```python
from build123d import *

# Parameters (mm, degrees)
SKETCH2_W           = 57
SKETCH2_H           = 120.75
SKETCH2_W_2         = 51
SKETCH2_H_2         = 114.75
BOSS_EXTRUDE1_DEPTH = 75
SKETCH3_W           = 57
SKETCH3_H           = 120.75
BOSS_EXTRUDE2_DEPTH = 3
SKETCH4_W           = 78
SKETCH4_H           = 57
BOSS_EXTRUDE3_DEPTH = 5
SKETCH6_R           = 2.675
CUT_EXTRUDE2_DEPTH  = 10
CUT_EXTRUDE3_DEPTH  = 58
BOSS_EXTRUDE4_REACH = 59
CUT_EXTRUDE7_DEPTH  = 126.75
SKETCH18_R          = 1.75
SKETCH18_W          = 28.5
SKETCH18_H          = 55
CUT_EXTRUDE8_DEPTH  = 10
BOSS_EXTRUDE6_DEPTH = 5
CUT_EXTRUDE9_DEPTH  = 5
CHAMFER1_SIZE       = 2


with BuildPart() as part:
    # Sketch2 → Boss-Extrude1 (new body)
    with BuildSketch(Plane(origin=(0, 0, 0), x_dir=(0, 0, -1), z_dir=(1, 0, 0))):
        with Locations((2.896243414, -39.494242434)):
            Rectangle(SKETCH2_W, SKETCH2_H)
        with Locations((2.896243414, -39.494242434)):
            Rectangle(SKETCH2_W_2, SKETCH2_H_2, mode=Mode.SUBTRACT)
    extrude(amount=BOSS_EXTRUDE1_DEPTH)

    # Sketch3 → Boss-Extrude2 (add)
    with BuildSketch(Plane.ZY):
        with Locations((-2.896243414, -39.494242434)):
            Rectangle(SKETCH3_W, SKETCH3_H)
    extrude(amount=BOSS_EXTRUDE2_DEPTH)

    # Sketch4 → Boss-Extrude3 (add)
    with BuildSketch(Plane(origin=(0, 20.880757566, 0), x_dir=(1, 0, 0), z_dir=(0, 1, 0))):
        with Locations((36, 2.896243414)):
            Rectangle(SKETCH4_W, SKETCH4_H)
    extrude(amount=BOSS_EXTRUDE3_DEPTH)

    # Sketch6 → Cut-Extrude2 (cut)
    with BuildSketch(Plane(origin=(0, 25.880757566, 0), x_dir=(1, 0, 0), z_dir=(0, 1, 0))):
        with Locations((36, 18.896243414)):
            Circle(SKETCH6_R)
        with Locations((36, -13.103756586)):
            Circle(SKETCH6_R)
    extrude(amount=-CUT_EXTRUDE2_DEPTH, mode=Mode.SUBTRACT)

    # Sketch8 → Cut-Extrude3 (cut, through all)
    with BuildSketch(Plane(origin=(0, 0, -31.396243414), x_dir=(-1, 0, 0), z_dir=(0, 0, -1))):
        Polygon((3, -99.869242434), (3, -79.869242434), (-17, -99.869242434), align=None)
    extrude(amount=-CUT_EXTRUDE3_DEPTH, mode=Mode.SUBTRACT)

    # Sketch9 → Boss-Extrude4 (add, up to next)
    with BuildSketch(Plane.XY.offset(25.603756586), mode=Mode.PRIVATE) as boss_extrude4_sk1:
        Polygon((-3, -79.869242434), (17, -99.869242434), (21.242640687, -99.869242434), (-3, -75.626601747), align=None)
    boss_extrude4_tool1 = extrude(boss_extrude4_sk1.sketch, amount=-BOSS_EXTRUDE4_REACH, mode=Mode.PRIVATE) - part.part
    add(boss_extrude4_tool1.solids().sort_by_distance((8.094564, -88.774678, 25.603757))[0])

    # Sketch15 → Cut-Extrude7 (cut, through all)
    with BuildSketch(Plane.XZ.offset(99.869242434)):
        with BuildLine():
            Line((62.625, 7.226342188), (62.625, 11.976342188))
            ThreePointArc((62.625, 11.976342188), (65, 14.351342188), (67.375, 11.976342188))
            Line((67.375, 11.976342188), (67.375, 7.226342188))
            ThreePointArc((67.375, 7.226342188), (65, 4.851342188), (62.625, 7.226342188))
        make_face()
        with BuildLine():
            Line((62.625, -17.72757696), (62.625, -12.97757696))
            ThreePointArc((62.625, -12.97757696), (65, -10.60257696), (67.375, -12.97757696))
            Line((67.375, -12.97757696), (67.375, -17.72757696))
            ThreePointArc((67.375, -17.72757696), (65, -20.10257696), (62.625, -17.72757696))
        make_face()
    extrude(amount=-CUT_EXTRUDE7_DEPTH, mode=Mode.SUBTRACT)

    # Sketch18 → Cut-Extrude8 (cut)
    with BuildSketch(Plane.ZY.offset(3)):
        with Locations((-22.896243414, -14.119242434)):
            Circle(SKETCH18_R)
        with Locations((17.103756586, -14.119242434)):
            Circle(SKETCH18_R)
        with Locations((-2.896243414, -14.119242434)):
            Rectangle(SKETCH18_W, SKETCH18_H)
    extrude(amount=-CUT_EXTRUDE8_DEPTH, mode=Mode.SUBTRACT)

    # Sketch21 → Boss-Extrude6 (add)
    with BuildSketch(Plane(origin=(0, 0, 0), x_dir=(0, 0, -1), z_dir=(1, 0, 0))):
        with BuildLine():
            Line((22.896243414, -19.869242434), (28.646243414, -19.869242434))
            Line((28.646243414, -19.869242434), (28.646243414, -8.369242434))
            Line((28.646243414, -8.369242434), (22.896243414, -8.369242434))
            ThreePointArc((22.896243414, -8.369242434), (17.146243414, -14.119242434), (22.896243414, -19.869242434))
        make_face()
        Polygon((19.518744339, -14.119242434), (21.207493877, -11.194242434), (24.584992952, -11.194242434), (26.273742489, -14.119242434), (24.584992952, -17.044242434), (21.207493877, -17.044242434), align=None, mode=Mode.SUBTRACT)
        with BuildLine():
            Line((-17.103756586, -19.869242434), (-22.853756586, -19.869242434))
            Line((-22.853756586, -19.869242434), (-22.853756586, -8.369242434))
            Line((-22.853756586, -8.369242434), (-17.103756586, -8.369242434))
            ThreePointArc((-17.103756586, -8.369242434), (-11.353756586, -14.119242434), (-17.103756586, -19.869242434))
        make_face()
        Polygon((-15.415007048, -11.194242434), (-18.792506123, -11.194242434), (-20.481255661, -14.119242434), (-18.792506123, -17.044242434), (-15.415007048, -17.044242434), (-13.726257511, -14.119242434), align=None, mode=Mode.SUBTRACT)
    extrude(amount=BOSS_EXTRUDE6_DEPTH)

    # Sketch22 → Cut-Extrude9 (cut)
    with BuildSketch(Plane.XZ.offset(-17.880757566)):
        Polygon((40.820874748, -18.896243414), (38.410437374, -14.721243414), (33.589562626, -14.721243414), (31.179125252, -18.896243414), (33.589562626, -23.071243414), (38.410437374, -23.071243414), align=None)
        Polygon((38.410437374, 17.278756586), (40.820874748, 13.103756586), (38.410437374, 8.928756586), (33.589562626, 8.928756586), (31.179125252, 13.103756586), (33.589562626, 17.278756586), align=None)
    extrude(amount=-CUT_EXTRUDE9_DEPTH, mode=Mode.SUBTRACT)

    # Chamfer1
    chamfer1_edges = [part.edges().sort_by_distance(p)[0] for p in [
        (-3, -26.994242434, -31.396243414),
        (-3, 25.880757566, -2.896243414),
        (-3, -26.994242434, 25.603756586),
    ]]
    chamfer(chamfer1_edges, length=CHAMFER1_SIZE)


solid = part.part
```
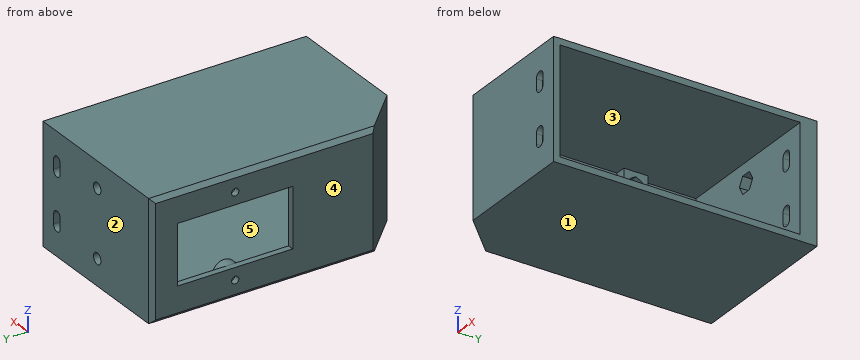
Geometry: final body of the model. Coordinates: model frame, mm. Face numbers are marked on the shaded views. A direction names the side the tool comes from. Give positions to 0.01 mm unless a question says otherwise; leave off trailing zeros. Order: outer loops, then holes, each group sorted by start corner. A loop starts at its lowest first (then second) coordinate and runs counter-clockwise, first axis right, second up. Notation, with made-up numbers: M 18,31 L 24,31 A24 ccw 24,66 Z; hole C -17.75,-28 d7. An arc over 180 degrees is marked long. Answer as CSV lines item,"result". Start each with the question number.
1) First-contact query: P1, Ø3.5, axis at y = -98, z = 9.5, coming from the -X side; P2, Ø4.5, axis at y = -14.12, z = 17.1, coming from the +X side; P3, Ø6.5, axis at y = -14.5, z = -24.5, coming from the +X side. Flat tips, straight axial feed; report the tip coordinate or a pass-through.
2) Cut plane A-A (x = 36). Output: boundary loops of the cut face in (y, z), then the cut area to 3 significant figures.
3) Cut plane C-C (x = 65). Output: boundary loops of the cut face in (y, z).
4) Line query: line 1 (Z direction, x = 36, y = 25); line 2 (Y direction, x = 67, z = -22.5); line 3 (Z direction, x = 3, y = -65). Output: solid intervals per line, ascending. Write a range as from..to.
5) Cut plane B-B (y = 2.5). Output: boundary loops of the cut face in (x, z).
6) Cut plane D-D (y = -62). Output: boundary loops of the cut face in (x, z).
7) Set-up query: the marked faces 4 and 5. Return all of +Z, -Z, +X, -X, +Y, -Y with unobstructed straight access to the full face (end or side cutting, diameter ignored); none if empty.
8) Mould query, pull axis Z, two halves, no side actions, for the marked faces 1, 2 and 3. Classes: +Z half, -Z half, draft (parallel to the pull), parting line (faces both ways), or undercut.
Findings below:
1,P1,"stops at x = 13.38"
1,P2,"stops at x = 0"
1,P3,"stops at x = 5"
2,outline,"M -99.87,-31.4 L 25.88,-31.4 L 25.88,-21.57 L 22.88,-21.57 L 22.88,-23.07 L 17.88,-23.07 L 17.88,-28.4 L -96.87,-28.4 L -96.87,22.6 L 17.88,22.6 L 17.88,17.28 L 22.88,17.28 L 22.88,15.78 L 25.88,15.78 L 25.88,25.6 L -99.87,25.6 Z; M 17.88,-14.72 L 22.88,-14.72 L 22.88,-16.22 L 25.88,-16.22 L 25.88,10.43 L 22.88,10.43 L 22.88,8.93 L 17.88,8.93 Z"
2,area,"1,200 mm²"
3,outline,"M -99.87,-31.4 L 25.88,-31.4 L 25.88,-20.1 L 17.88,-20.1 L 17.88,-28.4 L -96.87,-28.4 L -96.87,-20.1 L -99.87,-20.1 Z; M -99.87,-10.6 L -96.87,-10.6 L -96.87,4.85 L -99.87,4.85 Z; M -99.87,14.35 L -96.87,14.35 L -96.87,22.6 L 17.88,22.6 L 17.88,14.35 L 25.88,14.35 L 25.88,25.6 L -99.87,25.6 Z; M 17.88,-10.6 L 25.88,-10.6 L 25.88,4.85 L 17.88,4.85 Z"
4,line 1,"z = -31.4..-21.57, -16.22..10.43, 15.78..25.6"
4,line 2,"y = -99.87..-96.87, 17.88..25.88"
4,line 3,"z = -31.4..-28.4, 22.6..25.6"
5,outline,"M -3,-29.4 L -1,-31.4 L 75,-31.4 L 75,-28.4 L 0,-28.4 L 0,-17.15 L -3,-17.15 Z; M -3,11.35 L 0,11.35 L 0,22.6 L 75,22.6 L 75,25.6 L -1,25.6 L -3,23.6 Z"
6,outline,"M -3,-29.4 L -1,-31.4 L 75,-31.4 L 75,-28.4 L 0,-28.4 L 0,22.6 L 75,22.6 L 75,25.6 L -1,25.6 L -3,23.6 Z"
7,face 4,"+Z, -Z, -X, +Y, -Y"
7,face 5,"+X"
8,face 1,"-Z half"
8,face 2,"draft"
8,face 3,"undercut"
